```python
from build123d import *

# Parameters (mm, degrees)
SKETCH_1_R      = 4.75
EXTRUDE_1_DEPTH = 1.3
SKETCH_2_R      = 2.5
EXTRUDE_2_DEPTH = 16
CHAMFER_1_SIZE  = 0.5
FILLET_1_SIZE   = 1
FILLET_1_SIZE_2 = 2


with BuildPart() as part:
    # 草图1 → 凸台-拉伸1 (new body)
    with BuildSketch(Plane(origin=(0, 0, 0), x_dir=(1, 0, 0), z_dir=(0, 1, 0))):
        with Locations(Location((0, 0, 0), (0, 0, 270))):
            Circle(SKETCH_1_R)
        Polygon((0, -1.732050808), (1.5, -0.866025404), (1.5, 0.866025404), (0, 1.732050808), (-1.5, 0.866025404), (-1.5, -0.866025404), align=None, mode=Mode.SUBTRACT)
    extrude(amount=EXTRUDE_1_DEPTH)

    # 草图2 → 凸台-拉伸2 (add)
    with BuildSketch(Plane(origin=(0, 1.3, 0), x_dir=(1, 0, 0), z_dir=(0, 1, 0))):
        with Locations(Location((0, 0, 0), (0, 0, 270))):
            Circle(SKETCH_2_R)
    extrude(amount=EXTRUDE_2_DEPTH)

    # 倒角1
    chamfer_1_edges = [part.edges().sort_by_distance(p)[0] for p in [
        (0, 17.3, -2.5),
    ]]
    chamfer(chamfer_1_edges, length=CHAMFER_1_SIZE)

    # 圆角1
    # an asymmetric fillet: 2, 1 mm, written as the material it takes off along each edge
    with BuildSketch(Plane(origin=(0, 0, 0), x_dir=(0, 0, 1), z_dir=(-1, 0, 0))) as fillet_1_piece_1:
        with BuildLine():
            Bezier((4.75, FILLET_1_SIZE), (4.75, 0), (4.75 - FILLET_1_SIZE_2, 0), weights=[1, 0.707106781, 1])
            Line((4.75 - FILLET_1_SIZE_2, 0), (4.75, 0))
            Line((4.75, 0), (4.75, FILLET_1_SIZE))
        make_face()
    revolve(axis=Axis((0, 0, 0), (0, 1, 0)), mode=Mode.SUBTRACT)


solid = part.part
```
Part model, mm, in its own coordinate system. A direction names the side the tool comes from. Coordinates: 2 decimals unless noted, no trailing zeros. Loops run counter-clockwise (first coordinate to the right, second up) from the corner with the lowest first, then second, coordinate; pieces in that order, holes last. Notation, with made-up numbers: (2, 17) - (48, 17) arc R22 cw to (48, 32) - close; hole circle Ø11 at (1, 18.25). An arc over 180 degrees is marked (long way). Write item = value, one per line. Start each with the question number.
Item 1: Cut at A-A, the plane y = 14.25. Give the cut face in (x, z), and give its area (3 significant figures).
Item 2: Wall check: L1, parallel to X at y = 5, z = 0; L2, parallel to X at y = 7, z = -1.5; L3, parallel to Y at x = 4, z = -1.25. Give the ranges that are in metal, low to high. Write a range as from..to.
Item 3: 3-axis set-ups, long thin cutter, end or side, ignore diameter. For faces 1 (the cylindrical face through (-2.89, 1.15, -3.77)), 2 (the flat face through (1.5, 1, 0)), 3 (the flat face through (-2, 1.3, 2)): which of +Z, -Z, +X, -X, +Y, -Y reach the whole face in a straight line?
Item 4: Mould opens along Z. For faces 4 (the cylindrical face through (-2.44, 8.94, -0.54)), 5 (the flat face through (-0.76, 0.641, 1.293)), 6 (the flat face through (0, 17.3, 0)) say: released by +Z, released by -Z, zero draft, split by the parting line, or undercut.
Item 5: Flat gauge pins, fed straight in: pin 1 Ø1.5 at (x, z) = (2.5, -3.5) entering from +Y; pin 2 Ø0.6 at (y, z) = (1, 0.5) entering from +X; pin 3 Ø4 at (y, z) = (8.5, -2) entering from +X; pin 4 Ø3.5 at (x, z) = (0, -0.5) entering from -Y. Where does each tip first touch, or does it go through?
The answers:
q1.outline = circle Ø5 at (0, 0)
q1.area = 19.6 mm2
q2.L1 = -2.5..2.5
q2.L2 = -2..2
q2.L3 = 0.31..1.3
q3.face_1 = +Y, -Y
q3.face_2 = -Y
q3.face_3 = +Y
q4.face_4 = split by the parting line
q4.face_5 = undercut
q4.face_6 = zero draft
q5.pin_1 = 1.3
q5.pin_2 = 4.75
q5.pin_3 = 2.5
q5.pin_4 = 0
